```python
from build123d import *

# Parameters (mm, degrees)
F0_R     = 8
F0_R_2   = 2.5
F1_DEPTH = 11
F0_R_3   = 9
F2_DEPTH = 0.5
F3_START = 10.5
F3_DEPTH = 0.5


with BuildPart() as f1:
    # F0 (on Top) → F1 (new body)
    with BuildSketch(Plane.XY):
        Circle(F0_R)
        Circle(F0_R_2, mode=Mode.SUBTRACT)
    extrude(amount=F1_DEPTH)

    # F0 (on Top) → F2 (join)
    with BuildSketch(Plane.XY):
        Circle(F0_R_3)
        Circle(F0_R, mode=Mode.SUBTRACT)
    extrude(amount=F2_DEPTH)

    # F0 (on Top) → F3 (join)
    with BuildSketch(Plane.XY.offset(F3_START)):
        Circle(F0_R_3)
        Circle(F0_R, mode=Mode.SUBTRACT)
    extrude(amount=F3_DEPTH)


solid = f1.part
```
The listing builds one solid part. Answer for the finished solid, in the listing's coordinates (mm). Round coordinates to 2 decimals unless told otherwise and drop trailing zeros. Order: outer loops, then holes, each group sorted by start corner. A loop starts at its lowest first (then second) coordinate and runs counter-clockwise, first axis right, second up. Notation, with made-up numbers: (66.25, 47.25) -> (86.25, 47.25) arc R23 ccw to (86.25, 66.25) -> close; hole circle Ø8 at (-32.5, 2.25). An arc over 180 degrees is marked (long way). Answer as CSV lines item,"result".
Q1. Given pin 1 (1 mm diameter, centred on y = 4.5, z = 5.5, fed in from -X); pin 2 (4 mm diameter, centred on y = -3.5, z = 1.5, fed in from -X); pin 3 (1.5 mm diameter, centred on x = 6.5, z = 3.5, fed in from +Y), each flat-ended and moving along its own axis, determine where each tip first touches the part or whether it passes through.
Computed values:
pin 1,"stops at x = -6.93"
pin 2,"stops at x = -8.82"
pin 3,"stops at y = 5.56"
Q2. A cutting plane is placed at A-A on y = 0. Determine the outline of the cut face in (x, z), plus the area to 3 significant figures.
Computed values:
outline,"(-9, 0) -> (-2.5, 0) -> (-2.5, 11) -> (-9, 11) -> (-9, 10.5) -> (-8, 10.5) -> (-8, 0.5) -> (-9, 0.5) -> close; (2.5, 0) -> (9, 0) -> (9, 0.5) -> (8, 0.5) -> (8, 10.5) -> (9, 10.5) -> (9, 11) -> (2.5, 11) -> close"
area,"123 mm^2"
Q3. For a pull along Z with two mould halves and no side action, classify faces 1 (the flat face through (2, -2, 11)), 2 (the cylindrical face through (-1.73, -7.81, 5.43)), 3 (the cylindrical face through (-1.172, 8.923, 0.246)), 4 (the flat face through (2, -2, 0)) as +Z half, -Z half, draft (parallel to the pull), parting line (faces both ways), or undercut.
Computed values:
face 1,"+Z half"
face 2,"undercut"
face 3,"draft"
face 4,"-Z half"
Q4. A cutting plane is placed at C-C on z = 5.5. Determine the outline of the cut face in (x, y), plus the area to 3 significant figures.
Computed values:
outline,"circle Ø16 at (0, 0); hole circle Ø5 at (0, 0)"
area,"181 mm^2"
Q5. A cutting plane is placed at D-D on y = -4.75. Determine the outline of the cut face in (x, z), plus the area to 3 significant figures.
Computed values:
outline,"(-7.64, 0) -> (7.64, 0) -> (7.64, 0.5) -> (6.44, 0.5) -> (6.44, 10.5) -> (7.64, 10.5) -> (7.64, 11) -> (-7.64, 11) -> (-7.64, 10.5) -> (-6.44, 10.5) -> (-6.44, 0.5) -> (-7.64, 0.5) -> close"
area,"144 mm^2"
Q6. Consider line 1 (Z direction, x = -7.25, y = 5); line 2 (Y direction, x = 0, z = 5.75); line 3 (X direction, y = 1.75, z = 9.5). Determine where each line is inside the solid, lowest interval first. Write a range as from..to.
Computed values:
line 1,"z = 0..0.5, 10.5..11"
line 2,"y = -8..-2.5, 2.5..8"
line 3,"x = -7.81..-1.79, 1.79..7.81"
